Part model, mm, in its own coordinate system. Coordinates: 2 decimals unless noted, no trailing zeros. Loops run counter-clockwise (first coordinate to the right, second up) from the corner with the lowest first, then second, coordinate; pieces in that order, holes last. Notation, with made-up numbers: M 11,-12.75 L 47,-12.75 A23 ccw 47,23.25 Z; hole C -35,57.25 d8. An arc over 180 degrees is marked long. Use a Markdown table: item, result. Add a question column.
1) Wall check: probe 1 along X at (y, z) = (8, 2.75); probe 2 along Y at (x, z) = (-19, 3.75); probe 3 along Y at (x, z) = (13, 4). Give the ranges that are in metal, low to high. Write a range as from..to.
2) Band-saw the part on C-C (z = 5). State how many separate pieces and enclosed holes the cut face has, plus the area to 3 significant figures.
3) Pull direction X, two halves, no side cores. Call faces 1 (the flat face through (25, 0, 4)), 2 (the cylindrical face through (17.5, 8.07, 3.6)), 3 (the flat face through (0, 0, 0)), 4 (the flat face through (-25, 0, 4)): released by +X, released by -X, zero draft, split by the parting line, or undercut.
4) Band-saw the part on B-B (x = -19). List the corners of the cut face in (y, z), plus the area to 3 significant figures.
5) Pin check, flat tip, straight feed: pin 1 Ø1.8 at (x, y) = (-19, 8) entering from +Z. Stop position of the tip, or through.
6) Band-saw the part on A-A (y = 13). List the corners of the cut face in (x, z).
from build123d import *

# Parameters (mm, degrees)
SKETCH1_W               = 50
SKETCH1_H               = 40
SKETCH1_R               = 1.5
BOSS_EXTRUDE1_DEPTH     = 7.3
CUT_EXTRUDE1_DEPTH      = 33.837326322
CUT_EXTRUDE1_DEPTH_BACK = 33.837326322
SKETCH2_R               = 1.5


with BuildPart() as part:
    # Sketch1 → Boss-Extrude1 (new body)
    with BuildSketch(Plane.XY):
        Rectangle(SKETCH1_W, SKETCH1_H)
        with Locations((-13, 13)):
            Circle(SKETCH1_R, mode=Mode.SUBTRACT)
        with Locations(Location((13, 13, 0), (0, 0, 180))):
            Circle(SKETCH1_R, mode=Mode.SUBTRACT)
        with Locations((13, -13)):
            Circle(SKETCH1_R, mode=Mode.SUBTRACT)
        with Locations(Location((-13, -13, 0), (0, 0, 180))):
            Circle(SKETCH1_R, mode=Mode.SUBTRACT)
    extrude(amount=BOSS_EXTRUDE1_DEPTH)

    # Sketch2 → Cut-Extrude1 (cut, two sides: drawn at the far end of the back side and taken through both)
    with BuildSketch(Plane.XY.offset(7.3).offset(-CUT_EXTRUDE1_DEPTH_BACK)):
        with Locations((-19, 8)):
            Circle(SKETCH2_R)
        with Locations((19, 8)):
            Circle(SKETCH2_R)
        with Locations((19, -8)):
            Circle(SKETCH2_R)
        with Locations((-19, -8)):
            Circle(SKETCH2_R)
    extrude(amount=CUT_EXTRUDE1_DEPTH + CUT_EXTRUDE1_DEPTH_BACK, mode=Mode.SUBTRACT)


solid = part.part
Entries:
| question | item | result |
|---|---|---|
| 1 | probe 1 | -25..-20.5, -17.5..17.5, 20.5..25 |
| 1 | probe 2 | -20..-9.5, -6.5..6.5, 9.5..20 |
| 1 | probe 3 | -20..-14.5, -11.5..11.5, 14.5..20 |
| 2 | separate pieces | 1 |
| 2 | enclosed holes | 8 |
| 2 | area | 1,940 mm2 |
| 3 | face 1 | released by +X |
| 3 | face 2 | undercut |
| 3 | face 3 | zero draft |
| 3 | face 4 | released by -X |
| 4 | outline | M -20,0 L -9.5,0 L -9.5,7.3 L -20,7.3 Z; M -6.5,0 L 6.5,0 L 6.5,7.3 L -6.5,7.3 Z; M 9.5,0 L 20,0 L 20,7.3 L 9.5,7.3 Z |
| 4 | area | 248 mm2 |
| 5 | pin 1 | through |
| 6 | outline | M -25,0 L -14.5,0 L -14.5,7.3 L -25,7.3 Z; M -11.5,0 L 11.5,0 L 11.5,7.3 L -11.5,7.3 Z; M 14.5,0 L 25,0 L 25,7.3 L 14.5,7.3 Z |
